Study the drawing (mm; zero at the part's minimum x, y, z) and answer. Coordinates: 2 decimals unless noted, no trailing zeros. Loops run counter-clockwise (first coordinate to the right, second up) from the corner with the lowest first, then second, coordinate; pieces in that order, holes last. Notation, with made-up numbers: M -34,51 L -15,51 A17 ccw -15,60 Z; hole C 14,57.5 d1. An arc over 180 degrees is marked long. Use one line per item in the form item = value. Start each with the question number.
1. The part is cut by section B-B (z = 79.5). Give the vertices of the cut face in (x, y), plus the area to 3 significant figures.
2. The part is cut by section A-A (y = 3). Give the vertices of the cut face in (x, z) (1 decimal).
3. Find the intervals of material crossed by probe 1 along X at (y, z) = (3, 76); probe 2 along X at (y, z) = (3.25, 116), in increasing order. Write a range as [from, to].
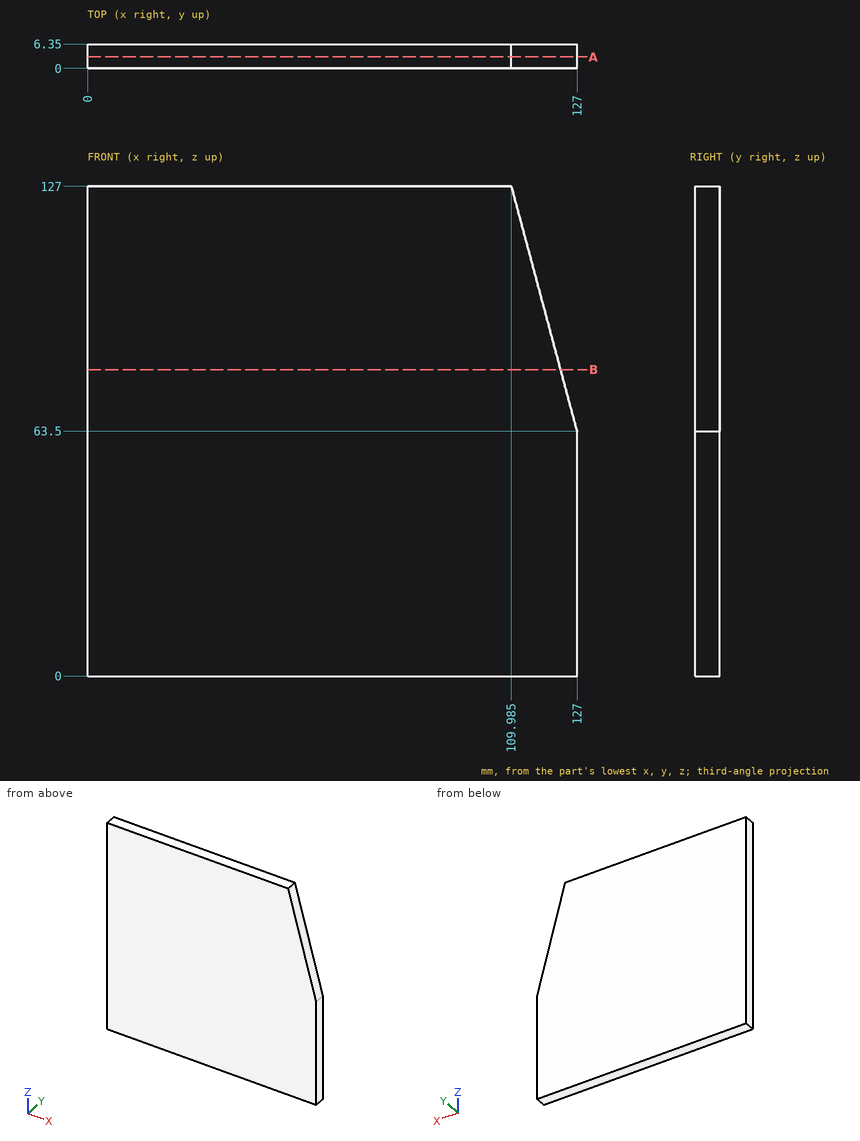
Computed values:
q1.outline = M 0,0 L 122.71,0 L 122.71,6.35 L 0,6.35 Z
q1.area = 779 mm²
q2.outline = M 0,0 L 127,0 L 127,63.5 L 110,127 L 0,127 Z
q3.probe_1 = [0, 123.65]
q3.probe_2 = [0, 112.93]
